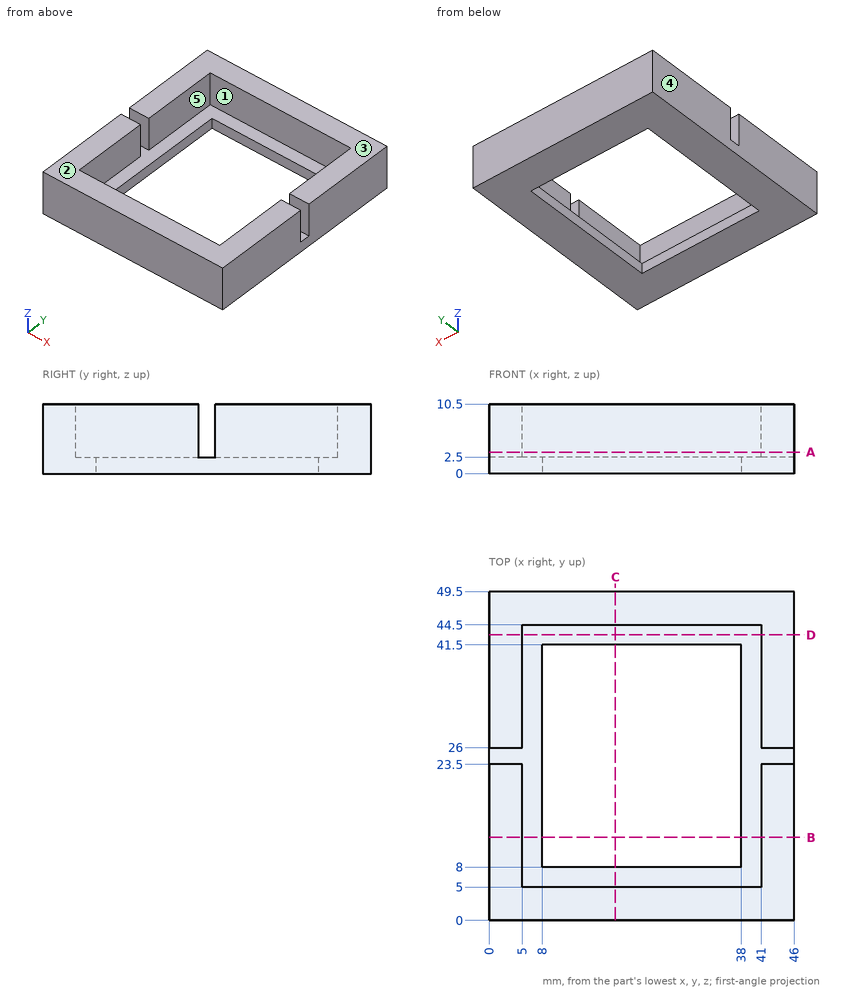
Could you check a few things on this drawing? It's one solid part, dimensions in mm from its lowest x, y, z. A direction names the side the tool comes from. Round coordinates to 2 decimals unless told otherwise and drop trailing zeros. Order: outer loops, then holes, each group sorted by start corner. A loop starts at its lowest first (then second) coordinate and runs counter-clockwise, first axis right, second up. Notation, with made-up numbers: M 53.25,-31.5 L 85.25,-31.5 A16 cw 85.25,-21.5 Z; hole C 55,-24 d4. An arc over 180 degrees is marked long. Return JSON: item names as keys, results as strings. Group by question number.
1. If we section it at C-C on x = 19: List the corners of the cut face in (y, z) for me.
2. Please list where these lines run through material, in increasing order: probe 1 along Y at (x, z) = (31, 9.25); probe 2 along Y at (x, z) = (28, 1); probe 3 along X at (y, z) = (43, 4.5).
3. If we section it at B-B on y = 12.5: List the corners of the cut face in (x, z) for me, then the cut area to 3 significant figures.
4. If we mould it in two halves opening along X, with no side actions, what happens to the marked faces 3, 4 and 5? For each: pulls with the +X half, pulls with the -X half, needs draft (parallel to the pull), parting line crosses it, or undercut.
5. If we section it at D-D on y = 43: List the corners of the cut face in (x, z) for me.
6. If we section it at A-A on z = 3.25: List the corners of the cut face in (x, y) for me, then the cut area to 3 significant figures.
7. I'm going to push flat-ended pins straight in: pin 1 Ø2 at (y, z) = (17.5, 1) entering from -X; pin 2 Ø1.5 at (x, y) = (31, 41.5) entering from +Z. Where does each tip first touch, or does it pass through?
8. On a 3-axis mill with a long thin cutter (end or side, diameter ignored), from which of +Z, -Z, +X, -X, +Y, -Y can I reach the whole of each face in a straight line? I mean the marked faces 1 and 2. Say none if no direction works.
Reply:
{
 "1": {"outline": "M 0,0 L 8,0 L 8,2.5 L 5,2.5 L 5,10.5 L 0,10.5 Z; M 41.5,0 L 49.5,0 L 49.5,10.5 L 44.5,10.5 L 44.5,2.5 L 41.5,2.5 Z"},
 "2": {"probe 1": "0 to 5, 44.5 to 49.5", "probe 2": "0 to 8, 41.5 to 49.5", "probe 3": "0 to 5, 41 to 46"},
 "3": {"outline": "M 0,0 L 8,0 L 8,2.5 L 5,2.5 L 5,10.5 L 0,10.5 Z; M 38,0 L 46,0 L 46,10.5 L 41,10.5 L 41,2.5 L 38,2.5 Z", "area": "120 mm^2"},
 "4": {"face 3": "needs draft", "face 4": "pulls with the -X half", "face 5": "undercut"},
 "5": {"outline": "M 0,0 L 46,0 L 46,10.5 L 41,10.5 L 41,2.5 L 5,2.5 L 5,10.5 L 0,10.5 Z"},
 "6": {"outline": "M 0,0 L 46,0 L 46,23.5 L 41,23.5 L 41,5 L 5,5 L 5,23.5 L 0,23.5 Z; M 0,26 L 5,26 L 5,44.5 L 41,44.5 L 41,26 L 46,26 L 46,49.5 L 0,49.5 Z", "area": "830 mm^2"},
 "7": {"pin 1": "x = 0", "pin 2": "z = 2.5"},
 "8": {"face 1": "+Z", "face 2": "+Z, +X, -X, +Y, -Y"}
}
